Build history of the part. All positions in model axes, mm. A direction names the side the tool comes from. Round coordinates to 2 decimals unless told otherwise and drop trailing zeros. Loops run counter-clockwise (first coordinate to the right, second up) from the corner with the lowest first, then second, coordinate; pieces in that order, holes last.
from build123d import *

# Parameters (mm, degrees)
BOSS_EXTRUDE1_DEPTH = 26.858
CUT_EXTRUDE1_REACH  = 113.995
SKETCH2_W           = 6.858
SKETCH2_H           = 50
CUT_EXTRUDE2_REACH  = 74.541
SKETCH3_R           = 1.55
FILLET1_R           = 5


with BuildPart() as part:
    # Sketch1 → Boss-Extrude1 (new body)
    with BuildSketch(Plane.XY):
        Polygon((-47.852923476, -42.680149177), (2.147076524, 27.319850823), (52.147076524, -42.680149177), align=None)
    extrude(amount=BOSS_EXTRUDE1_DEPTH)

    # Cut-Extrude1: up to this plane
    cut_extrude1_end = Plane(origin=(-47.852923476, -42.680149177, 26.858), z_dir=(0.8137334712067356, -0.5812381937190956, 0))
    # Sketch2 → Cut-Extrude1 (cut, up to the surface)
    with BuildSketch(Plane.ZY.offset(-52.147076524), mode=Mode.PRIVATE) as cut_extrude1_sk1:
        with Locations((13.429, 2.319850823)):
            Rectangle(SKETCH2_W, SKETCH2_H)
    cut_extrude1_tool1 = split(extrude(cut_extrude1_sk1.sketch, amount=CUT_EXTRUDE1_REACH, mode=Mode.PRIVATE), bisect_by=cut_extrude1_end, keep=Keep.BOTH, mode=Mode.PRIVATE)
    add(cut_extrude1_tool1.solids().sort_by_distance((52.147077, 2.319851, 13.429))[0], mode=Mode.SUBTRACT)

    # Cut-Extrude2: up to this face of the body (flat: up to its plane)
    cut_extrude2_end = Plane(part.part.faces().sort_by_distance((2.147076524, -19.346815843, 0))[0])
    # Sketch3 → Cut-Extrude2 (cut, up to the picked face)
    with BuildSketch(Plane.XY.offset(26.858), mode=Mode.PRIVATE) as cut_extrude2_sk1:
        with Locations((2.147076524, 6.819850823)):
            Circle(SKETCH3_R)
    cut_extrude2_tool1 = split(extrude(cut_extrude2_sk1.sketch, amount=-CUT_EXTRUDE2_REACH, mode=Mode.PRIVATE), bisect_by=cut_extrude2_end, keep=Keep.BOTH, mode=Mode.PRIVATE)
    add(cut_extrude2_tool1.solids().sort_by(Axis((2.147077, 6.819851, 26.858), (0, 0, -1)))[0], mode=Mode.SUBTRACT)

    # Fillet1
    fillet1_edges = [part.edges().sort_by_distance(p)[0] for p in [
        (2.147076524, 27.319850823, 5),
        (2.147076524, 27.319850823, 21.858),
    ]]
    fillet(fillet1_edges, radius=FILLET1_R)


solid = part.part
(1) Which spindle directions (+Z, -Z, +X, -X, +Y, -Y) get a long thin tool onto all of the face, cutting with end or side? Do faces 1 (the face through (3, -5, 16.858)), 2 (the face through (2.081, 23.717, 5.07)). Say none if no direction does.
Responses:
face 1: +X, -X, +Y
face 2: +Z, -Z, +Y
(2) Slice it at B-B on x = 31. List the corners of the cut face in (y, z).
Responses:
outline: (-42.68, 0) - (-13.07, 0) - (-13.07, 10) - (-22.68, 10) - (-22.68, 16.86) - (-13.07, 16.86) - (-13.07, 26.86) - (-42.68, 26.86) - close
(3) Probe line 1 (Z direction, x = 14, y = -5); line 2 (Y direction, x = 25, z = 11.5); line 3 (X direction, y = 6.5, z = 17.5). List the from-to ranges inside material, lowest first.
Responses:
line 1: z = 0 to 10, 16.86 to 26.86
line 2: y = -42.68 to -22.68
line 3: x = -12.72 to 0.63, 3.66 to 17.02
(4) Slice it at D-D on z = 18.25. List the corners of the cut face in (x, y).
Responses:
outline: (-47.85, -42.68) - (52.15, -42.68) - (6.22, 21.62) arc R5 ccw to (-1.92, 21.62) - close; hole circle Ø3.1 at (2.15, 6.82)
(5) Slice it at A-A on y = 18.5. List the corners of the cut face in (x, z).
Responses:
outline: (-4.15, 0) - (8.45, 0) - (8.45, 10) - (-4.15, 10) - close; (-4.15, 16.86) - (8.45, 16.86) - (8.45, 26.86) - (-4.15, 26.86) - close
(6) Slice it at C-C on z = 12. List the corners of the cut face in (x, y).
Responses:
outline: (-47.85, -42.68) - (52.15, -42.68) - (37.86, -22.68) - (-33.57, -22.68) - close
(7) Pin check, flat tips, straight feed: P1, Ø8, axis at y = 12, z = 22.5, coming from the +X side; P2, Ø1, axis at x = -6, z = 19, coming from the +Y side; P3, Ø10, axis at y = -21.5, z = 8.5, coming from the +X side. Stop position of each tip, or through.
Responses:
P1: stops at x = 15.95
P2: stops at y = 16.61
P3: stops at x = 40.59
(8) Pull direction Y, two halves, no side cores. Call faces 3 (the face through (3, -5, 10)), 4 (the face through (1.811, 5.307, 5.07)), 5 (the face through (1.811, 5.307, 21.928)), 6 (the face through (-25.21, -10.98, 7.27)): +Y half, -Y half, draft (parallel to the pull), parting line (faces both ways), or undercut.
Responses:
face 3: draft
face 4: undercut
face 5: undercut
face 6: +Y half
